```python
from build123d import *
from build123d.topology import SkipClean

# Parameters (mm, degrees)
SKETCH1_W          = 120
SKETCH1_H          = 25
BASE_DEPTH         = 5
CLIP_DEPTH         = 120
SKETCH3_R          = 1.5
SCREWHOLES_DEPTH   = 10
CLIPWALL_DEPTH     = 3
ROUNDEDCORNERS_R   = 1
SKETCH5_W          = 15.150992531
SKETCH5_H          = 29
FINGERGAP_DEPTH    = 15
FINGERGROOVE_R     = 5
CUT_EXTRUDE1_START = -2
SKETCH3_3_R        = 3
SKETCH3_3_R_2      = 1.5
CUT_EXTRUDE1_DEPTH = 5


with BuildPart() as part:
    # Sketch1 → Base (new body)
    with BuildSketch(Plane(origin=(0, 0, 0), x_dir=(0, 0, -1), z_dir=(1, 0, 0))):
        with Locations((60, 12.5)):
            Rectangle(SKETCH1_W, SKETCH1_H)
    extrude(amount=BASE_DEPTH)

    # Sketch2 → Clip (add)
    with BuildSketch(Plane.XY):
        with BuildLine():
            Line((25.150992531, 27), (7, 27))
            ThreePointArc((7, 27), (5.585786438, 26.414213562), (5, 25))
            Line((5, 25), (5, 12.5))
            ThreePointArc((5, 12.5), (12.740541767, 24.773008971), (27.150992531, 23.075468156))
            Line((27.150992531, 23.075468156), (27.150992531, 25))
            ThreePointArc((27.150992531, 25), (26.565206094, 26.414213562), (25.150992531, 27))
        make_face()
        with BuildLine():
            ThreePointArc((27.150992531, 1.924531844), (12.740541767, 0.226991029), (5, 12.5))
            Line((5, 12.5), (5, 0))
            ThreePointArc((5, 0), (5.585786438, -1.414213562), (7, -2))
            Line((7, -2), (25.150992531, -2))
            ThreePointArc((25.150992531, -2), (26.565206094, -1.414213562), (27.150992531, 0))
            Line((27.150992531, 0), (27.150992531, 1.924531844))
        make_face()
    extrude(amount=-CLIP_DEPTH)

    # Sketch3 → ScrewHoles (cut)
    with SkipClean():  # the faces are left unmerged after this step: merging them gives an invalid solid
        with BuildSketch(Plane.ZY):
            with Locations((-100, 12.5)):
                Circle(SKETCH3_R)
            with Locations((-20, 12.5)):
                Circle(SKETCH3_R)
        extrude(amount=-SCREWHOLES_DEPTH, mode=Mode.SUBTRACT)

    # Sketch4 → ClipWall (add)
    with SkipClean():  # the faces are left unmerged after this step: merging them gives an invalid solid
        with BuildSketch(Plane.XY):
            with BuildLine():
                ThreePointArc((10.354216867, 4.341136076), (7, 12.5), (10.354216867, 20.658863924))
                ThreePointArc((10.354216867, 20.658863924), (11.424450472, 22.274442864), (11.8, 24.175615615))
                Line((11.8, 24.175615615), (11.8, 24.277945491))
                ThreePointArc((11.8, 24.277945491), (5, 12.5), (11.8, 0.722054509))
                Line((11.8, 0.722054509), (11.8, 0.824384385))
                ThreePointArc((11.8, 0.824384385), (11.424450472, 2.725557136), (10.354216867, 4.341136076))
            make_face()
        clipwall = extrude(amount=-CLIPWALL_DEPTH)

    # Mirror1: ClipWall across plane
    with SkipClean():  # the faces are left unmerged after this step: merging them gives an invalid solid
        add(clipwall.mirror(Plane(origin=(0, 0, -60), x_dir=(1, 0, 0), z_dir=(0, 0, -1))))

    # RoundedCorners
    roundedcorners_edges = [part.edges().sort_by_distance(p)[0] for p in [
        (27.150992531, 23.075468156, -60),
        (27.150992531, 1.924531844, -60),
    ]]
    fillet(roundedcorners_edges, radius=ROUNDEDCORNERS_R)

    # Sketch5 → FingerGap (cut, symmetric)
    with BuildSketch(Plane(origin=(0, 0, -60), x_dir=(-1, 0, 0), z_dir=(0, 0, -1))):
        with Locations((-19.575496265, 12.5)):
            Rectangle(SKETCH5_W, SKETCH5_H)
    extrude(amount=FINGERGAP_DEPTH, both=True, mode=Mode.SUBTRACT)

    # FingerGroove
    # the kernel refuses this fillet: 5 mm, written as the material it takes off along each edge
    with BuildSketch(Plane(origin=(12, 0.608826803, -75), x_dir=(0, -1, 0), z_dir=(0, 0, 1))) as fingergroove_piece_1:
        with BuildLine():
            CenterArc((2.648427898, -5), FINGERGROOVE_R, 90, 51.416397028)
            ThreePointArc((-1.26006702, -1.88172043), (-0.590797761, -0.96713387), (0, 0))
            Line((0, 0), (2.648427898, 0))
        make_face()
    extrude(amount=30, mode=Mode.SUBTRACT)
    with BuildSketch(Plane(origin=(12, 24.391173197, -75), x_dir=(0, 1, 0), z_dir=(0, 0, 1))) as fingergroove_piece_2:
        with BuildLine():
            CenterArc((2.648427898, 5), FINGERGROOVE_R, 218.583602972, 51.416397028)
            ThreePointArc((-1.26006702, 1.88172043), (-0.590797761, 0.96713387), (0, 0))
            Line((0, 0), (2.648427898, 0))
        make_face()
    extrude(amount=30, mode=Mode.SUBTRACT)

    # Sketch3<3> → Cut-Extrude1 (cut)
    # profile 1 of 2: a face of its own
    with BuildSketch(Plane.ZY.offset(CUT_EXTRUDE1_START)):
        with Locations(Location((-100, 12.5, 0), (0, 0, 180))):
            Circle(SKETCH3_3_R)
        with Locations((-100, 12.5)):
            Circle(SKETCH3_3_R_2, mode=Mode.SUBTRACT)
    # profile 2 of 2: a face of its own
    with BuildSketch(Plane.ZY.offset(CUT_EXTRUDE1_START)):
        with Locations(Location((-20, 12.5, 0), (0, 0, 180))):
            Circle(SKETCH3_3_R)
        with Locations(Location((-20, 12.5, 0), (0, 0, 180))):
            Circle(SKETCH3_3_R_2, mode=Mode.SUBTRACT)
    extrude(amount=-CUT_EXTRUDE1_DEPTH, mode=Mode.SUBTRACT)


solid = part.part
```
Can you work these out from the model? Positions are in its coordinate system, mm. A direction names the side the tool comes from. Give positions to 0.01 mm unless a question says otherwise; leave off trailing zeros. Loops run counter-clockwise (first coordinate to the right, second up) from the corner with the lowest first, then second, coordinate; pieces in that order, holes last. Notation, with made-up numbers: M 21,-11.5 L 43,-11.5 A10 ccw 43,7.5 Z; hole C 66.25,20.5 d1. An arc over 180 degrees is marked long. Answer in a Markdown table with one row per item.
1. Suppose I cut it at A-A on z = -20. Write out the boundary of the cut face in (x, y) (3 decimals), plus the area to 3 significant figures.
Taken from the geometry:
| item | result |
|---|---|
| outline | M 0,0 L 5,0 A2 ccw 7,-2 L 25.151,-2 A2 ccw 27.151,0 L 27.151,0.004 A1 ccw 25.634,0.86 A13.6 cw 5.335,9.5 L 2,9.5 L 2,11 L 0,11 Z; M 0,14 L 2,14 L 2,15.5 L 5.335,15.5 A13.6 cw 25.634,24.14 A1 ccw 27.151,24.996 L 27.151,25 A2 ccw 25.151,27 L 7,27 A2 ccw 5,25 L 0,25 Z |
| area | 231 mm² |
2. Suppose I cut it at D-D on y = 18. Write out the boundary of the cut face in (x, z).
Taken from the geometry:
| item | result |
|---|---|
| outline | M 0,-120 L 8.39,-120 L 8.39,-117 L 6.16,-117 L 6.16,-3 L 8.39,-3 L 8.39,0 L 0,0 Z |
3. Which directions (+Z, -Z, +X, -X, +Y, -Y) give clear straight access to the entire face, cutting with the end or side of a thin tool? Please do faces 3 (the cylindrical face through (11.48, 24.82, -60.21)), 4 (the cylindrical face through (26.58, 26.4, -97.18)), 5 (the flat face through (2, 0, -59)), 6 (the cylindrical face through (7, 12.4, -1.5)), 7 (the flat face through (2, 25, -59)).
Taken from the geometry:
| item | result |
|---|---|
| face 3 | +X |
| face 4 | +Z, -Z, +X, +Y |
| face 5 | +Z, -Z, -X, -Y |
| face 6 | +Z, -Z, +X |
| face 7 | +Z, -Z, -X, +Y |
4. Suppose I cut it at B-B on x = 16.5. Write out the boundary of the cut face in (y, z).
Taken from the geometry:
| item | result |
|---|---|
| outline | M -2,-120 L -0.94,-120 L -0.94,-75 L -2,-75 Z; M -2,-45 L -0.94,-45 L -0.94,0 L -2,0 Z; M 25.94,-120 L 27,-120 L 27,-75 L 25.94,-75 Z; M 25.94,-45 L 27,-45 L 27,0 L 25.94,0 Z |
5. Suppose I cut it at C-C on z = -51. Write out the boundary of the cut face in (x, y).
Taken from the geometry:
| item | result |
|---|---|
| outline | M 0,0 L 5,0 A2 ccw 7,-2 L 12,-2 A5 ccw 10.12,1.87 A13.6 cw 10.12,23.13 A5 ccw 12,27 L 7,27 A2 ccw 5,25 L 0,25 Z |
6. Thinking about a two-plate mould opening in Z: for faces 1 (the cylindrical face through (7, 12.4, -118.5)), 2 (the cylindrical face through (0.99, 12.57, -21.5)), which applies, released by +Z, released by -Z, zero draft, split by the parting line, or undercut?
Taken from the geometry:
| item | result |
|---|---|
| face 1 | zero draft |
| face 2 | undercut |
7. For pin 1 Ø2 at (y, z) = (1, -69) entering from +X; pin 2 Ø1.2 at (x, y) = (20, 25) entering from +Z; pin 3 Ø1.8 at (y, z) = (13, -21.5) entering from +X; pin 4 Ø7 at (y, z) = (12.5, -100) entering from +X, each with a flat end and sliding along its axis, tell me the tip position at first contact or that it passes through.
Taken from the geometry:
| item | result |
|---|---|
| pin 1 | stops at x = 11.57 |
| pin 2 | passes through |
| pin 3 | stops at x = 2 |
| pin 4 | stops at x = 5.46 |
8. If I drill on line 1 along Z through (x, y) = (3.5, 12.5); line 2 along Y through (x, z) = (19.25, -89.5); line 3 along Y through (x, z) = (1, -100), over which ranges is the centre line in solid material (lowest first)?
Taken from the geometry:
| item | result |
|---|---|
| line 1 | z = -120 to -103, -97 to -23, -17 to 0 |
| line 2 | y = -2 to -1.08, 26.08 to 27 |
| line 3 | y = 0 to 11, 14 to 25 |
